Input: part model. Units: mm. Frame: model coordinates. A direction names the side the tool comes from. Give positions to 0.01 mm unless a question says otherwise; leave off trailing zeros. Order: outer loops, then holes, each group sorted by start corner. A loop starts at its lowest first (then second) coordinate and runs counter-clockwise, first axis right, second up. Notation, with made-up numbers: (62, 10.5) - (96, 10.5) arc R10 ccw to (96, 22.5) - close; hole circle Ø9 at (-8, 54.5). An arc over 180 degrees is marked (long way). Answer in a Markdown table with one row per item. Add a question column.
from build123d import *

# Parameters (mm, degrees)
F0_R     = 1.5
F1_DEPTH = 6
F2_R     = 2.5
F3_DEPTH = 1.5
F4_W     = 1
F4_H     = 1.5
F4_H_2   = 1
F4_W_2   = 1.5
F5_DEPTH = 1


# Not quite as in the source:
# - a fillet or chamfer that OpenCascade refuses, or shapes differently, is made with other operations: its cross-section is extruded or revolved along the edge and cut away or added


with BuildPart() as f1:
    # F0 (on Top) → F1 (new body)
    with BuildSketch(Plane.XY):
        Circle(F0_R)
    extrude(amount=F1_DEPTH)

    # F2 (on face) → F3 (join)
    with BuildSketch(Plane.XY.offset(6)):
        Circle(F2_R)
    extrude(amount=F3_DEPTH)

    # F4 (on face) → F5 (cut)
    with BuildSketch(Plane.XY.offset(7.5)):
        with Locations((0, 1.25)):
            Rectangle(F4_W, F4_H)
        Rectangle(F4_W, F4_H_2)
        with Locations((-1.25, 0)):
            Rectangle(F4_W_2, F4_H_2)
        with Locations((1.25, 0)):
            Rectangle(F4_W_2, F4_H_2)
        with Locations((0, -1.25)):
            Rectangle(F4_W, F4_H)
    extrude(amount=-F5_DEPTH, mode=Mode.SUBTRACT)

    # F6: fillet of radius 1 on 1 edges, made by hand

    # F6_s1 → F6_t2 (revolve, cut)
    with BuildSketch(Plane.XZ):
        with BuildLine():
            ThreePointArc((2.5, 6.5), (2.2071067812, 7.2071067812), (1.5, 7.5))
            Line((1.5, 7.5), (2.5, 7.5))
            Line((2.5, 7.5), (2.5, 6.5))
        make_face()
    revolve(axis=Axis((0, 0, 7.5), (0, 0, 1)), mode=Mode.SUBTRACT)

    # F7: fillet of radius 1 on 1 edges, made by hand

    # F7_s1 → F7_t2 (revolve, cut)
    with BuildSketch(Plane.XZ):
        with BuildLine():
            ThreePointArc((2.5, 6.5), (2.1339745962, 6.1339745962), (1.6339745962, 6))
            Line((1.6339745962, 6), (2.5, 6))
            Line((2.5, 6), (2.5, 6.5))
        make_face()
    revolve(axis=Axis((0, 0, 6), (0, 0, 1)), mode=Mode.SUBTRACT)


solid = f1.part
Q1. Access query for faces 4 (the flat face through (0.8, -0.8, 7.5)), 5 (the flat face through (0.5, 1, 7)). Directions: +Z, -Z, +X, -X, +Y, -Y. A direction counts if a zero-diameter tool reaches every point of the face in a straight line with its end or side. Return the directions, or none.
Q2. Section C-C, the plane z = 3.75. Return loops of the section in (x, y), then the cut area to 3 significant figures.
Q3. Contact query for flat-ended pins moving along their axis: P1, Ø0.7, axis at y = 0, z = 7, coming from the +X side; P2, Ø0.5, axis at x = -1.5, z = 7, coming from the -Y side; P3, Ø2, axis at y = 1.5, z = 6.5, coming from the -X side; P4, Ø1.6, axis at x = 0.5, y = 0.5, coming from the -Z side. Output: stop coordinate, or through.
Q4. Section A-A, the plane x = 0. Return loops of the section in (y, z), then the cut area to 3 significant figures.
Q5. Line query: probe 1 along Y at (x, z) = (-0.05, 0.5); probe 2 along Y at (x, z) = (-0.5, 2.25); probe 3 along Y at (x, z) = (0.75, 7). Output: solid intervals per line, ascending.
Q6. Pull-direction query (X, two-part tool) for faces 1 (the cylindrical face through (-1.5, 0.07, 2.96)), 2 (the flat face through (0.8, 0.9, 7.5)), 3 (the flat face through (0, -2, 7)); classes: +X half, -X half, draft (parallel to the pull), parting line (faces both ways), or undercut.
Computed:
| question | item | result |
|---|---|---|
| 1 | face 4 | +Z, +X, -X, +Y, -Y |
| 1 | face 5 | +Z |
| 2 | outline | circle Ø3 at (0, 0) |
| 2 | area | 7.07 mm^2 |
| 3 | P1 | stops at x = 2.49 |
| 3 | P2 | stops at y = -2.06 |
| 3 | P3 | stops at x = -2.45 |
| 3 | P4 | stops at z = 0 |
| 4 | outline | (-2.5, 6.5) arc R1 ccw to (-1.63, 6) - (-1.5, 6) - (-1.5, 0) - (1.5, 0) - (1.5, 6) - (1.63, 6) arc R1 ccw to (2.5, 6.5) arc R1 ccw to (2, 7.37) - (2, 6.5) - (-2, 6.5) - (-2, 7.37) arc R1 ccw to start |
| 4 | area | 20.9 mm^2 |
| 5 | probe 1 | y = -1.5 to 1.5 |
| 5 | probe 2 | y = -1.41 to 1.41 |
| 5 | probe 3 | y = -2.24 to -0.5, 0.5 to 2.24 |
| 6 | face 1 | parting line |
| 6 | face 2 | draft |
| 6 | face 3 | undercut |
